Autodesk Inventor part; units mm, degrees
ref_plane "YZ Plane" through (0, 0, 0) normal (1, 0, 0) x (0, 1, 0)
ref_plane "XZ Plane" through (0, 0, 0) normal (0, 1, 0) x (-1, 0, 0)
ref_plane "XY Plane" through (0, 0, 0) normal (0, 0, 1) x (1, 0, 0)
sketch "スケッチ1" plane through (0, 0, 0) normal (0, 0, 1) x (1, 0, 0)
  circle A0 centre (0, 0) radius 10
  dimension "d0" = 20
extrude "押し出し1" add sketch "スケッチ1" along normal blind 3
sketch "スケッチ5" plane through (0, 0, 3) normal (0, 0, 1) x (1, 0, 0)
  circle A0 centre (0, 7) radius 1
  circle A1 centre (0, 0) radius 10
  dimension "d30" = 2
  dimension "d77" = 0
  dimension "d78" = 7
hole "穴4" at (0, 7, 3) direction (0, 0, -1) diameter 1.5 end through all
sketch "スケッチ6" plane through (0, 0, 0) normal (0, 0, -1) x (-1, 0, 0)
  circle A0 centre (0, 0) radius 10
  circle A1 centre (0, 0) radius 4.05
  dimension "d66" = 8.1
hole "穴5" at (0, 0, 0) direction (0, 0, 1) diameter 8.1 end through all
sketch "スケッチ2" plane through (0, 0, 3) normal (0, 0, 1) x (1, 0, 0)
  circle A0 centre (0, 0) radius 10
  circle A1 centre (0, 0) radius 4.75
  dimension "d3" = 9.5
extrude "押し出し4" cut sketch "スケッチ2" against normal blind 0.5 contours A1
pattern_circular "円形状パターン3" count 8 over 360 about axis through (0, 0, 28.4429) along (0, 0, -1) of "穴4"
properties part number "03" material "アルミニウム 6061"
Input: part model. Units: mm. Frame: model coordinates. A direction names the side the tool comes from. Coordinates: 2 decimals unless noted, no trailing zeros. Loops run counter-clockwise (first coordinate to the right, second up) from the corner with the lowest first, then second, coordinate; pieces in that order, holes last. Notation, with made-up numbers: (29.25, -35.75) -> (49.25, -35.75) arc R25 ccw to (49.25, -23.75) -> close; hole circle Ø1 at (30.5, 41). An arc over 180 degrees is marked (long way). Use a Markdown table: item, result.
1) Cut plane A-A (y = 0). Return the cut outline in (x, z).
Results found:
| item | result |
|---|---|
| outline | (-10, 0) -> (-7.75, 0) -> (-7.75, 3) -> (-10, 3) -> close; (-6.25, 0) -> (-4.05, 0) -> (-4.05, 2.5) -> (-4.75, 2.5) -> (-4.75, 3) -> (-6.25, 3) -> close; (4.05, 0) -> (6.25, 0) -> (6.25, 3) -> (4.75, 3) -> (4.75, 2.5) -> (4.05, 2.5) -> close; (7.75, 0) -> (10, 0) -> (10, 3) -> (7.75, 3) -> close |
2) Pull-direction query (Y, two-part tool) for faces 3 (the cylindrical face through (-2.17, 9.76, 1.48)), 4 (the flat face through (4.3, 0.1, 0)), 5 (the cylindrical face through (7.75, 0.03, 1.48)); classes: released by +Y, released by -Y, zero draft, split by the parting line, or undercut.
Results found:
| item | result |
|---|---|
| face 3 | split by the parting line |
| face 4 | zero draft |
| face 5 | undercut |
3) Cut plane B-B (y = 7). Return the cut outline in (x, z).
Results found:
| item | result |
|---|---|
| outline | (-7.14, 0) -> (-0.75, 0) -> (-0.75, 3) -> (-7.14, 3) -> close; (0.75, 0) -> (7.14, 0) -> (7.14, 3) -> (0.75, 3) -> close |
4) Cut plane D-D (z = 0.3). Give the number of separate pieces and of enclosed holes in the cut face, then the cut area to 3 significant figures.
Results found:
| item | result |
|---|---|
| separate pieces | 1 |
| enclosed holes | 9 |
| area | 248 mm2 |
5) Material intervals for line 1 along X through (y, z) = (2.25, 1.55); line 2 along X through (y, z) = (-5.5, 1); line 3 along X through (y, z) = (-5.25, 1.85), sorted ascending. Write a range as from..to.
Results found:
| item | result |
|---|---|
| line 1 | x = -9.74..-3.37, 3.37..9.74 |
| line 2 | x = -8.35..-5.46, -4.44..4.44, 5.46..8.35 |
| line 3 | x = -8.51..-5.64, -4.26..4.26, 5.64..8.51 |
6) Contact query for a flat-ended pin moving along its axis: pin 1 (1 mm diameter, centred on y = -5, z = 1.5, fed in from -X). Output: stop coordinate, or through.
Results found:
| item | result |
|---|---|
| pin 1 | stops at x = -8.93 |
7) Access query for faces 1 (the flat face through (-2, 4, 2.5)), 2 (the cylindrical face through (5.54, -4.49, 1.48)). Directions: +Z, -Z, +X, -X, +Y, -Y. A direction counts if a zero-diameter tool reaches every point of the face in a straight line with its end or side. Return the directions, or none.
Results found:
| item | result |
|---|---|
| face 1 | +Z |
| face 2 | +Z, -Z |
